```python
from build123d import *

# Parameters (mm, degrees)
SKETCH1_W           = 39
SKETCH1_H           = 29
BOSS_EXTRUDE1_DEPTH = 1
SKETCH2_W           = 3
SKETCH2_H           = 15
BOSS_EXTRUDE2_DEPTH = 3
CHAMFER1_SIZE       = 1
CHAMFER2_SIZE       = 2
SKETCH3_W           = 11
SKETCH3_H           = 1
BOSS_EXTRUDE3_DEPTH = 0.5
FILLET1_R           = 0.5
CUT_EXTRUDE1_REACH  = 26.627
CUT_EXTRUDE2_REACH  = 26.627
SKETCH5_W           = 36
SKETCH5_H           = 3.5
CUT_EXTRUDE3_REACH  = 26.627
FILLET2_R           = 2


# Read off the part's stored shape, not the designer's step: Mirror1
# Some blends are built 0.0001 mm under size
with BuildPart() as part:
    # Sketch1 → Boss-Extrude1 (new body)
    with BuildSketch(Plane(origin=(0, 0, 0), x_dir=(1, 0, 0), z_dir=(0, 1, 0))):
        Rectangle(SKETCH1_W, SKETCH1_H)
    extrude(amount=BOSS_EXTRUDE1_DEPTH)

    # Sketch2 → Boss-Extrude2 (add)
    with BuildSketch(Plane(origin=(0, 1, 0), x_dir=(1, 0, 0), z_dir=(0, 1, 0))):
        with Locations((-16.9, 0)):
            Rectangle(SKETCH2_W, SKETCH2_H)
        with Locations((16.9, 0)):
            Rectangle(SKETCH2_W, SKETCH2_H)
    extrude(amount=BOSS_EXTRUDE2_DEPTH)

    # Chamfer1
    chamfer1_edges = [part.edges().sort_by_distance(p)[0] for p in [
        (0, 0, 14.5),
        (-19.5, 0, 0),
        (0, 0, -14.5),
        (19.5, 0, 0),
        (19.5, 0.5, 14.5),
        (-19.5, 0.5, 14.5),
        (-19.5, 0.5, -14.5),
        (19.5, 0.5, -14.5),
    ]]
    chamfer(chamfer1_edges, length=CHAMFER1_SIZE - 0.0001)  # a hair under: the kernel refuses the full size

    # Chamfer2
    chamfer2_edges = [part.edges().sort_by_distance(p)[0] for p in [
        (-15.4, 2.5, 7.5),
        (-15.4, 2.5, -7.5),
        (-16.9, 4, 7.5),
        (-15.4, 4, 0),
        (-16.9, 4, -7.5),
        (15.4, 2.5, -7.5),
        (15.4, 2.5, 7.5),
        (16.9, 4, -7.5),
        (15.4, 4, 0),
        (16.9, 4, 7.5),
    ]]
    chamfer(chamfer2_edges, length=CHAMFER2_SIZE)

    # Sketch3 → Boss-Extrude3 (add)
    with BuildSketch(Plane(origin=(18.4, 0, 0), x_dir=(0, 0, -1), z_dir=(1, 0, 0))):
        with Locations((0, 3.25)):
            Rectangle(SKETCH3_W, SKETCH3_H)
    extrude(amount=BOSS_EXTRUDE3_DEPTH)

    # Fillet1
    # the kernel refuses this fillet: 0.5 mm, written as the material it adds along each edge
    # the kernel refuses this fillet: 0.5 mm, written as the material it takes off along each edge
    with BuildSketch(Plane(origin=(18.4, 3.25, 5), x_dir=(1, 0, 0), z_dir=(0, 0, 1))) as fillet1_2_piece_1_section:
        Polygon((0, 0), (FILLET1_R * 1.02, 0), (FILLET1_R * 1.02, FILLET1_R * 1.02), (0, FILLET1_R * 1.02), align=None)
    fillet1_2_piece_1 = extrude(amount=FILLET1_R * 1.02, mode=Mode.PRIVATE)
    fillet1_2_piece_1 = fillet1_2_piece_1 - Plane(origin=(18.4, 3.25, 5), x_dir=(-0.7071067811865475, -0.7071067811865475, 0), z_dir=(0, 0, 1)) * Sphere(FILLET1_R, mode=Mode.PRIVATE)
    with BuildSketch(Plane(origin=(18.4, 3.25, 5), x_dir=(0, 0, 1), z_dir=(0, -1, 0))) as fillet1_2_piece_2_section:
        Polygon((0, 0), (FILLET1_R * 1.02, 0), (FILLET1_R * 1.02, -FILLET1_R * 1.02), (0, -FILLET1_R * 1.02), align=None)
    fillet1_2_piece_2 = extrude(amount=FILLET1_R * 1.02, mode=Mode.PRIVATE)
    fillet1_2_piece_2 = fillet1_2_piece_2 - Plane(origin=(18.4, 3.25, 5), x_dir=(-0.7071067811865475, 0, -0.7071067811865475), z_dir=(0, -1, 0)) * Sphere(FILLET1_R, mode=Mode.PRIVATE)
    with BuildSketch(Plane(origin=(18.4, 3.25, -5), x_dir=(0, -1, 0), z_dir=(0, 0, -1))) as fillet1_2_piece_3_section:
        Polygon((0, 0), (FILLET1_R * 1.02, 0), (FILLET1_R * 1.02, -FILLET1_R * 1.02), (0, -FILLET1_R * 1.02), align=None)
    fillet1_2_piece_3 = extrude(amount=FILLET1_R * 1.02, mode=Mode.PRIVATE)
    fillet1_2_piece_3 = fillet1_2_piece_3 - Plane(origin=(18.4, 3.25, -5), x_dir=(-0.7071067811865475, 0.7071067811865475, 0), z_dir=(0, 0, -1)) * Sphere(FILLET1_R, mode=Mode.PRIVATE)
    with BuildSketch(Plane(origin=(18.4, 3.25, -5), x_dir=(1, 0, 0), z_dir=(0, 0, -1))) as fillet1_2_piece_4_section:
        Polygon((0, 0), (FILLET1_R * 1.02, 0), (FILLET1_R * 1.02, -FILLET1_R * 1.02), (0, -FILLET1_R * 1.02), align=None)
    fillet1_2_piece_4 = extrude(amount=FILLET1_R * 1.02, mode=Mode.PRIVATE)
    fillet1_2_piece_4 = fillet1_2_piece_4 - Plane(origin=(18.4, 3.25, -5), x_dir=(-0.7071067811865475, -0.7071067811865475, 0), z_dir=(0, 0, -1)) * Sphere(FILLET1_R, mode=Mode.PRIVATE)
    with BuildSketch(Plane(origin=(18.9, 2.75, -5), x_dir=(-1, 0, 0), z_dir=(0, 0, 1)), Plane(origin=(18.9, 3.75, 5), x_dir=(-1, 0, 0), z_dir=(0, 0, -1))) as fillet1_2_piece_5:
        with BuildLine():
            CenterArc((FILLET1_R, -FILLET1_R), FILLET1_R, 90, 90)
            Line((0, -FILLET1_R), (0, 0))
            Line((0, 0), (FILLET1_R, 0))
        make_face()
    fillet1_2_piece_5_solid = extrude(amount=10, mode=Mode.PRIVATE)
    add([fillet1_2_piece_1, fillet1_2_piece_2, fillet1_2_piece_3, fillet1_2_piece_4, fillet1_2_piece_5_solid], mode=Mode.SUBTRACT)

    # Mirror1 outline → Mirror1 (revolve)
    with BuildSketch(Plane(origin=(-18.4, 3.25, 0), x_dir=(1, 0, 0), z_dir=(0, -1, 0))):
        with BuildLine():
            Line((0, 5.5), (0, -5.5))
            ThreePointArc((0, -5.5), (0.353553391, -5.353553391), (0.5, -5))
            Line((0.5, -5), (0.5, 5))
            ThreePointArc((0.5, 5), (0.353553391, 5.353553391), (0, 5.5))
        make_face()
    revolve(axis=Axis((-18.4, 3.25, 0), (0, 0, 1)))

    # Sketch4 → Cut-Extrude1 (cut, up to next)
    with BuildSketch(Plane.XZ, mode=Mode.PRIVATE) as cut_extrude1_sk1:
        with BuildLine():
            Line((9, 7.6), (-9, 7.6))
            ThreePointArc((-9, 7.6), (-10.5, 9.1), (-9, 10.6))
            Line((-9, 10.6), (9, 10.6))
            ThreePointArc((9, 10.6), (10.5, 9.1), (9, 7.6))
        make_face()
    cut_extrude1_tool1 = extrude(cut_extrude1_sk1.sketch, amount=-CUT_EXTRUDE1_REACH, mode=Mode.PRIVATE) & part.part
    add(cut_extrude1_tool1.solids().sort_by_distance((0, 0, 9.1))[0], mode=Mode.SUBTRACT)

    # Sketch5 → Cut-Extrude2 (cut, up to next)
    with BuildSketch(Plane(origin=(0, 0, 0), x_dir=(-1, 0, 0), z_dir=(0, -1, 0)), mode=Mode.PRIVATE) as cut_extrude2_sk1:
        with Locations((0, 11.25)):
            Rectangle(SKETCH5_W, SKETCH5_H)
    cut_extrude2_tool1 = extrude(cut_extrude2_sk1.sketch, amount=-CUT_EXTRUDE2_REACH, mode=Mode.PRIVATE) & part.part
    add(cut_extrude2_tool1.solids().sort_by_distance((0, 0, -11.25))[0], mode=Mode.SUBTRACT)

    # Sketch6 → Cut-Extrude3 (cut, up to next)
    with BuildSketch(Plane.XZ, mode=Mode.PRIVATE) as cut_extrude3_sk1:
        with BuildLine():
            Line((-6, -7.5), (-6, -9.5))
            Line((-6, -9.5), (-1, -9.5))
            Line((-1, -9.5), (-1, -7.5))
            ThreePointArc((-1, -7.5), (-3.5, -5), (-6, -7.5))
        make_face()
    cut_extrude3_tool1 = extrude(cut_extrude3_sk1.sketch, amount=-CUT_EXTRUDE3_REACH, mode=Mode.PRIVATE) & part.part
    add(cut_extrude3_tool1.solids().sort_by_distance((-3.5, 0, -7.478975))[0], mode=Mode.SUBTRACT)

    # Fillet2
    fillet2_edges = [part.edges().sort_by_distance(p)[0] for p in [
        (-6, 0.5, -9.5),
        (-1, 0.5, -9.5),
    ]]
    fillet(fillet2_edges, radius=FILLET2_R - 0.0001)  # a hair under: the kernel refuses the full size


solid = part.part
```
Verification items for the finished model (mm, model axes). A direction names the side the tool comes from. Coordinates: 2 decimals unless noted, no trailing zeros. Return JSON: item names as keys, results as strings.
(1) Mould release check, pull along X, two halves, no side actions. Record for faces 6 (the flat face through (-17.9, 1.5, 7.5)), 7 (the flat face through (16.4, 1.5, -6.5)), 8 (the flat face through (-18.4, 2, 0)): pulls with the +X half, pulls with the -X half, needs draft (parallel to the pull), parting line crosses it, or undercut.
Filled sheet:
{"face 6": "needs draft", "face 7": "undercut", "face 8": "pulls with the -X half"}
(2) Access from +Z, -Z, +X, -X, +Y, -Y to the whole of each face (thin tool, end or side, straight path). Record for faces 1 (the flat face through (15.4, 1.5, 0.1)), 2 (the flat face through (16.8, 2.8, -6.1)), 3 (the flat face through (17.9, 3, 6.5)), 4 (the flat face through (-16.8, 2.8, 6.1)), 5 (the flat face through (0.3, 0.5, -13)).
Filled sheet:
{"face 1": "+Z, -Z, +Y", "face 2": "-Z, +Y", "face 3": "+Z, +X, -X, +Y", "face 4": "+Z, +Y", "face 5": "+Y, -Y"}
(3) Section check B-B, the plane x = -3.5. Give the number of separate pieces and of enclosed holes in the cut face, and give its area (3 significant figures).
Filled sheet:
{"separate pieces": "3", "enclosed holes": "0", "area": "17.0 mm^2"}
(4) Thickness scan on line 1 along Z through (x, y) = (3, 0.35); line 2 along X through (y, z) = (1.3, 4.75); line 3 along Y through (x, z) = (10.5, 11.75). Record the ranges inside material, lowest first.
Filled sheet:
{"line 1": "z = -13.85 to -13, -9.5 to 7.6, 10.6 to 13.85", "line 2": "x = -18.4 to -15.4, 15.4 to 18.4", "line 3": "y = 0 to 1"}
(5) Go/stop test with flat-tipped pins: pin 1 (0.8 mm diameter, centred on x = -12.5, y = 0.5, fed in from -Z); pin 2 (0.5 mm diameter, centred on x = 3, y = 0.5, fed in from +Z); pin 3 (1.1 mm diameter, centred on x = 18, y = 1.5, fed in from +Z). Record where each tip stops, or that it passes through.
Filled sheet:
{"pin 1": "stops at z = -14.4", "pin 2": "stops at z = 14.25", "pin 3": "stops at z = 14.5"}
